For this review, take the finished solid that the model builds, in its own axes (mm). A direction names the side the tool comes from. Round coordinates to 2 decimals unless told otherwise and drop trailing zeros. Write each loop counter-clockwise with the first axis right and the second up, starting at its lowest first coordinate (ties: lowest second). Pieces come first, ordered by that corner, then holes. Notation, with made-up numbers: (-32, 8) -> (0, 8) arc R27 ccw to (0, 42) -> close; hole circle Ø10 at (-1.5, 63). An arc over 180 degrees is marked (long way). Answer in a Markdown table with one row per item.
from build123d import *

# Parameters (mm, degrees)
F1_DEPTH = 20
F2_DEPTH = 1
F3_START = 19
F3_DEPTH = 1


with BuildPart() as f1:
    # F0 (on Top) → F1 (new body)
    with BuildSketch(Plane.XY):
        with BuildLine():
            ThreePointArc((-9, 0), (0, 9), (9, 0))
            ThreePointArc((9, 0), (8.89226485, -1.388389656), (8.5716387029, -2.7435396748))
            Line((8.5716387029, -2.7435396748), (8.5716387029, -12.3096307803))
            ThreePointArc((8.5716387029, -12.3096307803), (13.2961381714, -6.9435372634), (15, 0))
            ThreePointArc((15, 0), (-7.0204907429, 13.2556670797), (-8.4283612971, -12.4081717366))
            Line((-8.4283612971, -12.4081717366), (-8.4283612971, -3.1563785967))
            ThreePointArc((-8.4283612971, -3.1563785967), (-8.8559373212, -1.6038622644), (-9, 0))
        make_face()
    extrude(amount=F1_DEPTH)

    # F0 (on Top) → F2 (join)
    with BuildSketch(Plane.XY):
        with BuildLine():
            ThreePointArc((15, 0), (13.2961381714, -6.9435372634), (8.5716387029, -12.3096307803))
            Line((8.5716387029, -12.3096307803), (8.5716387029, -12.9142173571))
            ThreePointArc((8.5716387029, -12.9142173571), (13.6585211479, -7.3276735771), (15.5, 0))
            ThreePointArc((15.5, 0), (-7.4030534205, 13.6178118673), (-8.4283612971, -13.0081791902))
            Line((-8.4283612971, -13.0081791902), (-8.4283612971, -12.4081717366))
            ThreePointArc((-8.4283612971, -12.4081717366), (-7.0204907429, 13.2556670797), (15, 0))
        make_face()
    extrude(amount=F2_DEPTH)

    # F0 (on Top) → F3 (join)
    with BuildSketch(Plane.XY.offset(F3_START)):
        with BuildLine():
            ThreePointArc((15, 0), (13.2961381714, -6.9435372634), (8.5716387029, -12.3096307803))
            Line((8.5716387029, -12.3096307803), (8.5716387029, -12.9142173571))
            ThreePointArc((8.5716387029, -12.9142173571), (13.6585211479, -7.3276735771), (15.5, 0))
            ThreePointArc((15.5, 0), (-7.4030534205, 13.6178118673), (-8.4283612971, -13.0081791902))
            Line((-8.4283612971, -13.0081791902), (-8.4283612971, -12.4081717366))
            ThreePointArc((-8.4283612971, -12.4081717366), (-7.0204907429, 13.2556670797), (15, 0))
        make_face()
    extrude(amount=F3_DEPTH)


solid = f1.part
1) Consider section B-B on z = 5.75. State the section outline as (x, y) points, then the cut area to 3 significant figures.
Solved:
| item | result |
|---|---|
| outline | (-8.43, -12.41) -> (-8.43, -3.16) arc R9 cw (long way) to (8.57, -2.74) -> (8.57, -12.31) arc R15 ccw (long way) to start |
| area | 337 mm² |
2) Consider section C-C on x = 0. State the section outline as (y, z) points.
Solved:
| item | result |
|---|---|
| outline | (9, 0) -> (15.5, 0) -> (15.5, 1) -> (15, 1) -> (15, 19) -> (15.5, 19) -> (15.5, 20) -> (9, 20) -> close |
3) Consider section A-A on y = 6.5. State the section outline as (x, z) points, then the cut area to 3 significant figures.
Solved:
| item | result |
|---|---|
| outline | (-14.07, 0) -> (-6.22, 0) -> (-6.22, 20) -> (-14.07, 20) -> (-14.07, 19) -> (-13.52, 19) -> (-13.52, 1) -> (-14.07, 1) -> close; (6.22, 0) -> (14.07, 0) -> (14.07, 1) -> (13.52, 1) -> (13.52, 19) -> (14.07, 19) -> (14.07, 20) -> (6.22, 20) -> close |
| area | 294 mm² |
4) Consider section D-D on y = -10. State the section outline as (x, z) points, then the cut area to 3 significant figures.
Solved:
| item | result |
|---|---|
| outline | (-11.84, 0) -> (-8.43, 0) -> (-8.43, 20) -> (-11.84, 20) -> (-11.84, 19) -> (-11.18, 19) -> (-11.18, 1) -> (-11.84, 1) -> close; (8.57, 0) -> (11.84, 0) -> (11.84, 1) -> (11.18, 1) -> (11.18, 19) -> (11.84, 19) -> (11.84, 20) -> (8.57, 20) -> close |
| area | 110 mm² |
5) For faces 1 (the flat face through (-6, 14, 19)), 2 (the flat face through (-8.428, -8, 10)), 3 (the flat face through (0, 11, 20)), list the 3-axis set-ups (+Z, -Z, +X, -X, +Y, -Y) from which the entire face can be reached by the end or side of a thin tool; tool diameter is ignored.
Solved:
| item | result |
|---|---|
| face 1 | none |
| face 2 | +Z, -Z, -Y |
| face 3 | +Z, +X, -X, +Y, -Y |
6) For line 1 (X direction, y = -4.5, z = 5.5); line 2 (Z direction, x = -13.5, y = -7.25); line 3 (X direction, y = 6.25, z = 18.25), list the stretches that pass through material, from the lowest coordinate up. Write a range as [from, to].
Solved:
| item | result |
|---|---|
| line 1 | [-14.31, -8.43], [8.57, 14.31] |
| line 2 | [0, 1], [19, 20] |
| line 3 | [-13.64, -6.48], [6.48, 13.64] |
7) Clearance check with flat-ended pins moving along their axes: pin 1 Ø2 at (y, z) = (10, 12) entering from +X; pin 2 Ø3 at (y, z) = (-6, 6) entering from +X; pin 3 Ø10 at (y, z) = (-5.5, 13.5) entering from +X. State where each tip first meets the part, or that it passes through.
Solved:
| item | result |
|---|---|
| pin 1 | x = 12 |
| pin 2 | x = 14.31 |
| pin 3 | x = 14.99 |
8) Mouldability with a two-part tool opening along Z and no side actions: class faces 4 (the flat face through (0, 11, 0)), 5 (the flat face through (8.572, -8, 10)), 6 (the flat face through (-6, 14, 1)) as pulls with the +Z half, pulls with the -Z half, needs draft (parallel to the pull), parting line crosses it, or undercut.
Solved:
| item | result |
|---|---|
| face 4 | pulls with the -Z half |
| face 5 | needs draft |
| face 6 | undercut |
